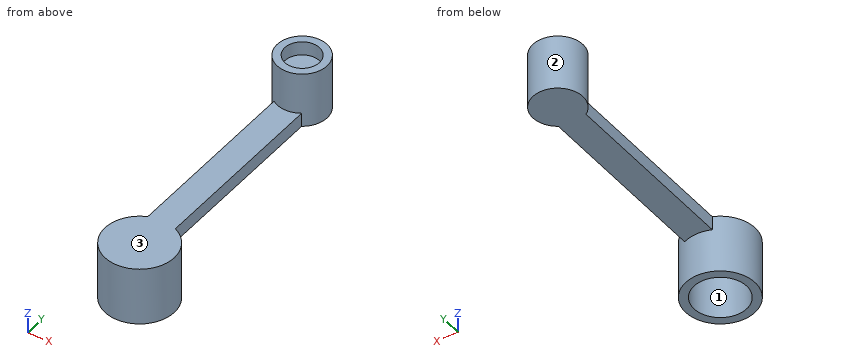
from build123d import *

# Parameters (mm, degrees)
EXTRUDE_1_DEPTH     = 1
SKETCH_2_R          = 1.8
EXTRUDE_2_DEPTH     = 4
SKETCH_3_R          = 1.25
CUT_EXTRUDE_1_DEPTH = 1
SKETCH_4_R          = 2.5
EXTRUDE_3_DEPTH     = 4.2
SKETCH_5_R          = 1.9
CUT_EXTRUDE_2_DEPTH = 4


with BuildPart() as part:
    # 草图1 → 凸台-拉伸1 (new body)
    with BuildSketch(Plane.XY):
        with BuildLine():
            Line((-1, 0), (-1, 17))
            ThreePointArc((-1, 17), (0, 18), (1, 17))
            Line((1, 17), (1, 0))
            ThreePointArc((1, 0), (0, -1), (-1, 0))
        make_face()
    extrude(amount=EXTRUDE_1_DEPTH)

    # 草图2 → 凸台-拉伸2 (add)
    with BuildSketch(Plane.XY):
        with Locations((0, 17)):
            Circle(SKETCH_2_R)
    extrude(amount=EXTRUDE_2_DEPTH)

    # 草图3 → 切除-拉伸1 (cut)
    with BuildSketch(Plane.XY.offset(4)):
        with Locations((0, 17)):
            Circle(SKETCH_3_R)
    extrude(amount=-CUT_EXTRUDE_1_DEPTH, mode=Mode.SUBTRACT)

    # 草图4 → 凸台-拉伸3 (add)
    with BuildSketch(Plane.XY.offset(1)):
        Circle(SKETCH_4_R)
    extrude(amount=-EXTRUDE_3_DEPTH)

    # 草图5 → 切除-拉伸2 (cut)
    with BuildSketch(Plane(origin=(0, 0, -3.2), x_dir=(-1, 0, 0), z_dir=(0, 0, -1))):
        Circle(SKETCH_5_R)
    extrude(amount=-CUT_EXTRUDE_2_DEPTH, mode=Mode.SUBTRACT)


solid = part.part
Read the model definition and answer for the solid it produces. Units are mm, in the model's axes. Face numbers are marked on the shaded views. Coordinates: 2 decimals unless noted, no trailing zeros. Loops run counter-clockwise (first coordinate to the right, second up) from the corner with the lowest first, then second, coordinate; pieces in that order, holes last. Notation, with made-up numbers: (34, 43) -> (77, 43) arc R25 ccw to (77, 63) -> close; hole circle Ø6 at (52.25, 55). An arc over 180 degrees is marked (long way). Answer in a Markdown table with one row per item.
Item 1: Each of these flat-tipped pins is pushed along its axis until it touches: P1, Ø1, axis at x = 1.5, z = -1, coming from the -Y side; P2, Ø2, axis at x = 1, y = 8, coming from the -Z side; P3, Ø3, axis at x = 0, y = 17, coming from the +Z side; P4, Ø1, axis at y = 6.5, z = -1, coming from the +X side. Where does it stop, or does it pass through?
Returned:
| item | result |
|---|---|
| P1 | stops at y = -2.29 |
| P2 | stops at z = 0 |
| P3 | stops at z = 4 |
| P4 | passes through |
Item 2: A cutting plane is placed at B-B on x = 0. Determine the outline of the cut face in (y, z).
Returned:
| item | result |
|---|---|
| outline | (-2.5, -3.2) -> (-1.9, -3.2) -> (-1.9, 0.8) -> (1.9, 0.8) -> (1.9, -3.2) -> (2.5, -3.2) -> (2.5, 0) -> (18.8, 0) -> (18.8, 4) -> (18.25, 4) -> (18.25, 3) -> (15.75, 3) -> (15.75, 4) -> (15.2, 4) -> (15.2, 1) -> (-2.5, 1) -> close |
Item 3: For a pull along X with two mould halves and no side action, classify the marked faces 1, 2 and 3 as released by +X, released by -X, zero draft, split by the parting line, or undercut.
Returned:
| item | result |
|---|---|
| face 1 | undercut |
| face 2 | split by the parting line |
| face 3 | zero draft |
Item 4: Straight lines are drawn through the part: line 1 along Y through (x, z) = (0, -2.2); line 2 along Z through (x, y) = (0.2, 14.25); line 3 along Y through (x, z) = (1.3, 2). For each, find the intervals that lie inside material, in ascending order. Write a range as [from, to].
Returned:
| item | result |
|---|---|
| line 1 | y = [-2.5, -1.9], [1.9, 2.5] |
| line 2 | z = [0, 1] |
| line 3 | y = [15.76, 18.24] |
Item 5: A cutting plane is placed at A-A on z = -1.5. Determine the outline of the cut face in (x, y).
Returned:
| item | result |
|---|---|
| outline | circle Ø5 at (0, 0); hole circle Ø3.8 at (0, 0) |
Item 6: A cutting plane is placed at D-D on y = 17. Determine the outline of the cut face in (x, z).
Returned:
| item | result |
|---|---|
| outline | (-1.8, 0) -> (1.8, 0) -> (1.8, 4) -> (1.25, 4) -> (1.25, 3) -> (-1.25, 3) -> (-1.25, 4) -> (-1.8, 4) -> close |
Item 7: A cutting plane is placed at C-C on y = 0. Determine the outline of the cut face in (x, z), plus the area to 3 significant figures.
Returned:
| item | result |
|---|---|
| outline | (-2.5, -3.2) -> (-1.9, -3.2) -> (-1.9, 0.8) -> (1.9, 0.8) -> (1.9, -3.2) -> (2.5, -3.2) -> (2.5, 1) -> (-2.5, 1) -> close |
| area | 5.80 mm^2 |
